from build123d import *

# Parameters (mm, degrees)
SKETCH1_W                    = 66.76
SKETCH1_H                    = 61.76
BOSS_EXTRUDE3_DEPTH          = 4
SKETCH2_R                    = 3.45
SKETCH2_R_2                  = 1.55
BOSS_EXTRUDE4_DEPTH          = 10
SKETCH3_R                    = 1.5
CUT_EXTRUDE1_DEPTH           = 3
CUT_EXTRUDE1_DRAFT           = 3
CUT_EXTRUDE1_PROFILE_2_DEPTH = 3
CUT_EXTRUDE1_PROFILE_2_DRAFT = 3
CUT_EXTRUDE1_PROFILE_3_DEPTH = 3
CUT_EXTRUDE1_PROFILE_3_DRAFT = 3
CUT_EXTRUDE1_PROFILE_4_DEPTH = 3
CUT_EXTRUDE1_PROFILE_4_DRAFT = 3
FILLET2_R                    = 2
FILLET1_R                    = 2
SKETCH5_R                    = 3.15
CUT_EXTRUDE2_DEPTH           = 2.5
CUT_EXTRUDE2_DRAFT           = -1
CUT_EXTRUDE2_PROFILE_2_DEPTH = 2.5
CUT_EXTRUDE2_PROFILE_2_DRAFT = -1
CUT_EXTRUDE2_PROFILE_3_DEPTH = 2.5
CUT_EXTRUDE2_PROFILE_3_DRAFT = -1
CUT_EXTRUDE2_PROFILE_4_DEPTH = 2.5
CUT_EXTRUDE2_PROFILE_4_DRAFT = -1


with BuildPart() as part:
    # Sketch1 → Boss-Extrude3 (new body)
    with BuildSketch(Plane(origin=(0, 0, 0), x_dir=(1, 0, 0), z_dir=(0, 1, 0))):
        with Locations((33.38, 30.88)):
            Rectangle(SKETCH1_W, SKETCH1_H)
    extrude(amount=-BOSS_EXTRUDE3_DEPTH)

    # Sketch2 → Boss-Extrude4 (add)
    # profile 1 of 4: a face of its own
    with BuildSketch(Plane(origin=(0, 0, 0), x_dir=(1, 0, 0), z_dir=(0, 1, 0))):
        with Locations(Location((58.76, 12.88, 0), (0, 0, 90))):
            Circle(SKETCH2_R)
        with Locations(Location((58.76, 12.88, 0), (0, 0, 270))):
            Circle(SKETCH2_R_2, mode=Mode.SUBTRACT)
    # profile 2 of 4: a face of its own
    with BuildSketch(Plane(origin=(0, 0, 0), x_dir=(1, 0, 0), z_dir=(0, 1, 0))):
        with Locations(Location((17.76, 12.88, 0), (0, 0, 90))):
            Circle(SKETCH2_R)
        with Locations(Location((17.76, 12.88, 0), (0, 0, 90))):
            Circle(SKETCH2_R_2, mode=Mode.SUBTRACT)
    # profile 3 of 4: a face of its own
    with BuildSketch(Plane(origin=(0, 0, 0), x_dir=(1, 0, 0), z_dir=(0, 1, 0))):
        with Locations(Location((58.76, 48.88, 0), (0, 0, 90))):
            Circle(SKETCH2_R)
        with Locations(Location((58.76, 48.88, 0), (0, 0, 90))):
            Circle(SKETCH2_R_2, mode=Mode.SUBTRACT)
    # profile 4 of 4: a face of its own
    with BuildSketch(Plane(origin=(0, 0, 0), x_dir=(1, 0, 0), z_dir=(0, 1, 0))):
        with Locations(Location((17.76, 48.88, 0), (0, 0, 90))):
            Circle(SKETCH2_R)
        with Locations(Location((17.76, 48.88, 0), (0, 0, 270))):
            Circle(SKETCH2_R_2, mode=Mode.SUBTRACT)
    extrude(amount=BOSS_EXTRUDE4_DEPTH)


with BuildPart() as cut_extrude1_tool:
    # Sketch3 → Cut-Extrude1 (with draft: the straight prism first)
    with BuildSketch(Plane(origin=(0, 0, 0), x_dir=(1, 0, 0), z_dir=(0, 1, 0))):
        with Locations((4.51, 57.25)):
            Circle(SKETCH3_R)
    extrude(amount=-CUT_EXTRUDE1_DEPTH)
    # Cut-Extrude1: the draft: its side faces are tilted about the plane it starts from
    cut_extrude1_sides = [cut_extrude1_tool.faces().sort_by_distance(p)[0] for p in [
        (3.01, -1.5, -57.25),
    ]]
    draft(cut_extrude1_sides, Plane(origin=(0, 0, 0), x_dir=(1, 0, 0), z_dir=(0, 1, 0)), CUT_EXTRUDE1_DRAFT)


with BuildPart() as part_1:
    add(part.part)

    # Cut-Extrude1: cut by cut_extrude1_tool
    add(cut_extrude1_tool.part, mode=Mode.SUBTRACT)


with BuildPart() as cut_extrude1_profile_2_tool:
    # Sketch3 → Cut-Extrude1 profile 2 (with draft: the straight prism first)
    with BuildSketch(Plane(origin=(0, 0, 0), x_dir=(1, 0, 0), z_dir=(0, 1, 0))):
        with Locations((62.25, 57.25)):
            Circle(SKETCH3_R)
    extrude(amount=-CUT_EXTRUDE1_PROFILE_2_DEPTH)
    # Cut-Extrude1 profile 2: the draft: its side faces are tilted about the plane it starts from
    cut_extrude1_profile_2_sides = [cut_extrude1_profile_2_tool.faces().sort_by_distance(p)[0] for p in [
        (60.75, -1.5, -57.25),
    ]]
    draft(cut_extrude1_profile_2_sides, Plane(origin=(0, 0, 0), x_dir=(1, 0, 0), z_dir=(0, 1, 0)), CUT_EXTRUDE1_PROFILE_2_DRAFT)


with BuildPart() as part_2:
    add(part_1.part)

    # Cut-Extrude1 profile 2: cut by cut_extrude1_profile_2_tool
    add(cut_extrude1_profile_2_tool.part, mode=Mode.SUBTRACT)


with BuildPart() as cut_extrude1_profile_3_tool:
    # Sketch3 → Cut-Extrude1 profile 3 (with draft: the straight prism first)
    with BuildSketch(Plane(origin=(0, 0, 0), x_dir=(1, 0, 0), z_dir=(0, 1, 0))):
        with Locations((62.25, 4.51)):
            Circle(SKETCH3_R)
    extrude(amount=-CUT_EXTRUDE1_PROFILE_3_DEPTH)
    # Cut-Extrude1 profile 3: the draft: its side faces are tilted about the plane it starts from
    cut_extrude1_profile_3_sides = [cut_extrude1_profile_3_tool.faces().sort_by_distance(p)[0] for p in [
        (60.75, -1.5, -4.51),
    ]]
    draft(cut_extrude1_profile_3_sides, Plane(origin=(0, 0, 0), x_dir=(1, 0, 0), z_dir=(0, 1, 0)), CUT_EXTRUDE1_PROFILE_3_DRAFT)


with BuildPart() as part_3:
    add(part_2.part)

    # Cut-Extrude1 profile 3: cut by cut_extrude1_profile_3_tool
    add(cut_extrude1_profile_3_tool.part, mode=Mode.SUBTRACT)


with BuildPart() as cut_extrude1_profile_4_tool:
    # Sketch3 → Cut-Extrude1 profile 4 (with draft: the straight prism first)
    with BuildSketch(Plane(origin=(0, 0, 0), x_dir=(1, 0, 0), z_dir=(0, 1, 0))):
        with Locations((4.51, 4.51)):
            Circle(SKETCH3_R)
    extrude(amount=-CUT_EXTRUDE1_PROFILE_4_DEPTH)
    # Cut-Extrude1 profile 4: the draft: its side faces are tilted about the plane it starts from
    cut_extrude1_profile_4_sides = [cut_extrude1_profile_4_tool.faces().sort_by_distance(p)[0] for p in [
        (3.01, -1.5, -4.51),
    ]]
    draft(cut_extrude1_profile_4_sides, Plane(origin=(0, 0, 0), x_dir=(1, 0, 0), z_dir=(0, 1, 0)), CUT_EXTRUDE1_PROFILE_4_DRAFT)


with BuildPart() as part_4:
    add(part_3.part)

    # Cut-Extrude1 profile 4: cut by cut_extrude1_profile_4_tool
    add(cut_extrude1_profile_4_tool.part, mode=Mode.SUBTRACT)

    # Fillet2
    fillet2_edges = [part_4.edges().sort_by_distance(p)[0] for p in [
        (0, -2, -61.76),
        (66.76, -2, -61.76),
        (66.76, -2, 0),
        (0, -2, 0),
    ]]
    fillet(fillet2_edges, radius=FILLET2_R)

    # Fillet1
    fillet1_edges = [part_4.edges().sort_by_distance(p)[0] for p in [
        (0, -4, -30.88),
        (33.38, -4, 0),
        (33.38, -4, -61.76),
        (66.76, -4, -30.88),
        (0.585786438, -4, -61.174213562),
        (66.174213562, -4, -61.174213562),
        (66.174213562, -4, -0.585786438),
        (0.585786438, -4, -0.585786438),
    ]]
    fillet(fillet1_edges, radius=FILLET1_R)


with BuildPart() as cut_extrude2_tool:
    # Sketch5 → Cut-Extrude2 (with draft: the straight prism first)
    with BuildSketch(Plane.XZ.offset(4)):
        with Locations((4.51, -4.51)):
            Circle(SKETCH5_R)
    extrude(amount=-CUT_EXTRUDE2_DEPTH)
    # Cut-Extrude2: the draft: its side faces are tilted about the plane it starts from
    cut_extrude2_sides = [cut_extrude2_tool.faces().sort_by_distance(p)[0] for p in [
        (1.36, -2.75, -4.51),
    ]]
    draft(cut_extrude2_sides, Plane.XZ.offset(4), CUT_EXTRUDE2_DRAFT)


with BuildPart() as part_5:
    add(part_4.part)

    # Cut-Extrude2: cut by cut_extrude2_tool
    add(cut_extrude2_tool.part, mode=Mode.SUBTRACT)


with BuildPart() as cut_extrude2_profile_2_tool:
    # Sketch5 → Cut-Extrude2 profile 2 (with draft: the straight prism first)
    with BuildSketch(Plane.XZ.offset(4)):
        with Locations((62.25, -4.51)):
            Circle(SKETCH5_R)
    extrude(amount=-CUT_EXTRUDE2_PROFILE_2_DEPTH)
    # Cut-Extrude2 profile 2: the draft: its side faces are tilted about the plane it starts from
    cut_extrude2_profile_2_sides = [cut_extrude2_profile_2_tool.faces().sort_by_distance(p)[0] for p in [
        (59.1, -2.75, -4.51),
    ]]
    draft(cut_extrude2_profile_2_sides, Plane.XZ.offset(4), CUT_EXTRUDE2_PROFILE_2_DRAFT)


with BuildPart() as part_6:
    add(part_5.part)

    # Cut-Extrude2 profile 2: cut by cut_extrude2_profile_2_tool
    add(cut_extrude2_profile_2_tool.part, mode=Mode.SUBTRACT)


with BuildPart() as cut_extrude2_profile_3_tool:
    # Sketch5 → Cut-Extrude2 profile 3 (with draft: the straight prism first)
    with BuildSketch(Plane.XZ.offset(4)):
        with Locations((62.25, -57.25)):
            Circle(SKETCH5_R)
    extrude(amount=-CUT_EXTRUDE2_PROFILE_3_DEPTH)
    # Cut-Extrude2 profile 3: the draft: its side faces are tilted about the plane it starts from
    cut_extrude2_profile_3_sides = [cut_extrude2_profile_3_tool.faces().sort_by_distance(p)[0] for p in [
        (59.1, -2.75, -57.25),
    ]]
    draft(cut_extrude2_profile_3_sides, Plane.XZ.offset(4), CUT_EXTRUDE2_PROFILE_3_DRAFT)


with BuildPart() as part_7:
    add(part_6.part)

    # Cut-Extrude2 profile 3: cut by cut_extrude2_profile_3_tool
    add(cut_extrude2_profile_3_tool.part, mode=Mode.SUBTRACT)


with BuildPart() as cut_extrude2_profile_4_tool:
    # Sketch5 → Cut-Extrude2 profile 4 (with draft: the straight prism first)
    with BuildSketch(Plane.XZ.offset(4)):
        with Locations((4.51, -57.25)):
            Circle(SKETCH5_R)
    extrude(amount=-CUT_EXTRUDE2_PROFILE_4_DEPTH)
    # Cut-Extrude2 profile 4: the draft: its side faces are tilted about the plane it starts from
    cut_extrude2_profile_4_sides = [cut_extrude2_profile_4_tool.faces().sort_by_distance(p)[0] for p in [
        (1.36, -2.75, -57.25),
    ]]
    draft(cut_extrude2_profile_4_sides, Plane.XZ.offset(4), CUT_EXTRUDE2_PROFILE_4_DRAFT)


with BuildPart() as part_8:
    add(part_7.part)

    # Cut-Extrude2 profile 4: cut by cut_extrude2_profile_4_tool
    add(cut_extrude2_profile_4_tool.part, mode=Mode.SUBTRACT)


solid = part_8.part
Could you check a few things on this model? Use its own coordinates, in mm. A direction names the side the tool comes from. Give positions to 0.01 mm unless a question says otherwise; leave off trailing zeros. Order: outer loops, then holes, each group sorted by start corner. A loop starts at its lowest first (then second) coordinate and runs counter-clockwise, first axis right, second up.
1. Will these pins go through, and if not, where does the flat tip stop? P1, Ø3, axis at x = 17.76, z = -12.88, coming from the +Y side; P2, Ø4, axis at x = 21.5, y = 7.5, coming from the -Z side; P3, Ø5, axis at x = 62.5, z = -4.5, coming from the -Y side.
2. Suppose I cut it at D-D (z = -33.5). List the corners of the cut face in (x, y) for me.
3. Suppose I cut it at B-B (x = 17.76). List the corners of the cut face in (y, z) for me.
4. Suppose I cut it at A-A (y = 5.75). List the corners of the cut face in (x, z) for me, plus the area to 3 significant figures.
5. Suppose I cut it at C-C (z = -48.88). List the corners of the cut face in (x, y) for me, plus the area to 3 significant figures.
6. I need wall thicknesses on L1, parallel to X at y = 5.5, z = -48.88; L2, parallel to X at y = 4.75, z = -10; L3, parallel to Y at x = 5, z = -54. Which ranges of each line are inside material? Lowest first, please.
7. For faces 1 (the flat face through (64, -1.5, -6)), 2 (the flat face through (16, 10, -13)), 3 (the flat face through (59, 0, -49)), which set-ups out of +Z, -Z, +X, -X, +Y, -Y let a thin tool reach every point of the face, with its end or its side?
Solved:
1. P1: stops at y = 0
1. P2: stops at z = -51.86
1. P3: stops at y = -1.5
2. outline: (0, -2) arc R2 ccw to (2, -4) - (64.76, -4) arc R2 ccw to (66.76, -2) - (66.76, 0) - (0, 0) - close
3. outline: (-4, -59.76) arc R2 ccw to (-2, -61.76) - (0, -61.76) - (0, -52.33) - (10, -52.33) - (10, -50.43) - (0, -50.43) - (0, -47.33) - (10, -47.33) - (10, -45.43) - (0, -45.43) - (0, -16.33) - (10, -16.33) - (10, -14.43) - (0, -14.43) - (0, -11.33) - (10, -11.33) - (10, -9.43) - (0, -9.43) - (0, 0) - (-2, 0) arc R2 ccw to (-4, -2) - close
4. outline: circle Ø6.9 at (17.76, -48.88); circle Ø6.9 at (17.76, -12.88); circle Ø6.9 at (58.76, -48.88); circle Ø6.9 at (58.76, -12.88); hole circle Ø3.1 at (17.76, -48.88); hole circle Ø3.1 at (17.76, -12.88); hole circle Ø3.1 at (58.76, -48.88); hole circle Ø3.1 at (58.76, -12.88)
4. area: 119 mm2
5. outline: (0, -2) arc R2 ccw to (2, -4) - (64.76, -4) arc R2 ccw to (66.76, -2) - (66.76, 0) - (62.21, 0) - (62.21, 10) - (60.31, 10) - (60.31, 0) - (57.21, 0) - (57.21, 10) - (55.31, 10) - (55.31, 0) - (21.21, 0) - (21.21, 10) - (19.31, 10) - (19.31, 0) - (16.21, 0) - (16.21, 10) - (14.31, 10) - (14.31, 0) - (0, 0) - close
5. area: 341 mm2
6. L1: x = 14.31 to 16.21, 19.31 to 21.21, 55.31 to 57.21, 60.31 to 62.21
6. L2: x = 15.86 to 19.66, 56.86 to 60.66
6. L3: y = -4 to 0
7. face 1: -Y
7. face 2: +Z, -Z, +X, -X, +Y
7. face 3: +Y
